Can you work these out from the model? Positions are in its coordinate system, mm. Face numbers are marked on the shaded views. A direction names the side the tool comes from. Round coordinates to 2 decimals unless told otherwise and drop trailing zeros. Loops run counter-clockwise (first coordinate to the right, second up) from the corner with the lowest first, then second, coordinate; pieces in that order, holes last. Notation, with made-up numbers: (51.5, 87) -> (81.5, 87) arc R22 ccw to (81.5, 106) -> close; hole circle Ø7 at (72.5, 9). An arc over 180 degrees is marked (long way). Write each question's results on one line, items separated by ' | '.
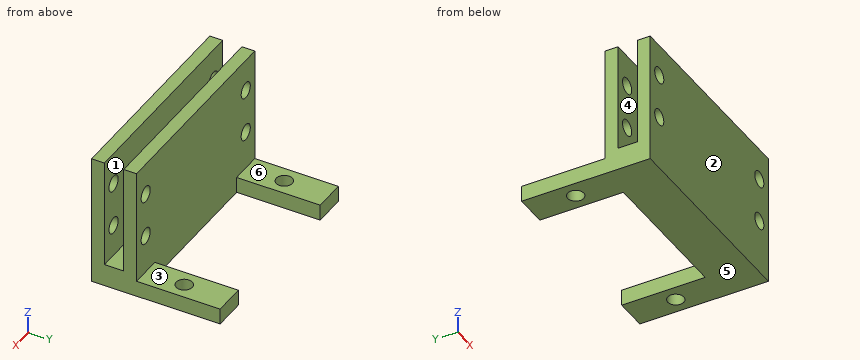
from build123d import *

# Parameters (mm, degrees)
SKETCH1_W               = 5
SKETCH1_H               = 13
SKETCH1_R               = 1.25
BOSS_EXTRUDE1_DEPTH     = 2.5
BOSS_EXTRUDE1_2_DEPTH   = 2.5
SKETCH1_5_W             = 32.5
SKETCH1_5_H             = 2
BOSS_EXTRUDE2_DEPTH     = 20.5
SKETCH1_6_W             = 32.5
SKETCH1_6_H             = 3
BOSS_EXTRUDE3_DEPTH     = 3.5
SKETCH2_R               = 1.25
CUT_EXTRUDE2_DEPTH      = 14
CUT_EXTRUDE2_DEPTH_BACK = 8


with BuildPart() as part:
    # Sketch1 → Boss-Extrude1 (new body)
    with BuildSketch(Plane.XY):
        with Locations((-13.75, 6.5)):
            Rectangle(SKETCH1_W, SKETCH1_H)
        with Locations((-13.75, 6)):
            Circle(SKETCH1_R, mode=Mode.SUBTRACT)
    extrude(amount=BOSS_EXTRUDE1_DEPTH)



with BuildPart() as body_2:
    # Sketch1 → Boss-Extrude1 2 (new body)
    with BuildSketch(Plane.XY):
        with Locations((13.75, 6.5)):
            Rectangle(SKETCH1_W, SKETCH1_H)
        with Locations((13.75, 6)):
            Circle(SKETCH1_R, mode=Mode.SUBTRACT)
    extrude(amount=BOSS_EXTRUDE1_2_DEPTH)


with BuildPart() as part_1:
    add(part.part)

    add(body_2.part)  # Boss-Extrude2 merges body 2
    # Sketch1<5> → Boss-Extrude2 (add)
    with BuildSketch(Plane.XY):
        with Locations((0, -1)):
            Rectangle(SKETCH1_5_W, SKETCH1_5_H)
        with Locations((0, -6)):
            Rectangle(SKETCH1_5_W, SKETCH1_5_H)
    extrude(amount=BOSS_EXTRUDE2_DEPTH)

    # Sketch1<6> → Boss-Extrude3 (add)
    with BuildSketch(Plane.XY):
        with Locations((0, -3.5)):
            Rectangle(SKETCH1_6_W, SKETCH1_6_H)
    extrude(amount=BOSS_EXTRUDE3_DEPTH)

    # Sketch2 → Cut-Extrude2 (cut, two sides)
    with BuildSketch(Plane(origin=(0, 0, 0), x_dir=(1, 0, 0), z_dir=(0, 1, 0))) as cut_extrude2_sk:
        with Locations((13.75, -8.5)):
            Circle(SKETCH2_R)
        with Locations((13.75, -15.5)):
            Circle(SKETCH2_R)
        with Locations((-13.75, -15.5)):
            Circle(SKETCH2_R)
        with Locations((-13.75, -8.5)):
            Circle(SKETCH2_R)
    extrude(amount=CUT_EXTRUDE2_DEPTH, mode=Mode.SUBTRACT)
    extrude(cut_extrude2_sk.sketch, amount=-CUT_EXTRUDE2_DEPTH_BACK, mode=Mode.SUBTRACT)


solid = part_1.part
1. Please list where these lines run through material, in increasing order: line 1 (Z direction, x = 13.75, y = -1); line 2 (Y direction, x = -8, z = 13.25); line 3 (Y direction, x = -13.75, z = 1). Write a range as from..to.
Final values:
line 1: 0..7.25, 9.75..14.25, 16.75..20.5 | line 2: -7..-5, -2..0 | line 3: -7..4.75, 7.25..13
2. If we section it at A-A (y = 9.75): List the corners of the cut face in (x, z) for me.
Final values:
outline: (-16.25, 0) -> (-11.25, 0) -> (-11.25, 2.5) -> (-16.25, 2.5) -> close; (11.25, 0) -> (16.25, 0) -> (16.25, 2.5) -> (11.25, 2.5) -> close
3. If we section it at C-C (x = 13.75): State how many separate pieces and enclosed holes the cut face has, then the cut area to 4 significant figures.
Final values:
separate pieces: 6 | enclosed holes: 0 | area: 98.75 mm2
4. We'd pull the mould along Y, two halves only. Please class the marked faces 1, 2, 3 and 4: pulls with the +Y half, pulls with the -Y half, needs draft (parallel to the pull), parting line crosses it, or undercut.
Final values:
face 1: undercut | face 2: pulls with the -Y half | face 3: needs draft | face 4: undercut
5. Will these pins go through, and if not, where does the flat tip stop? pin 1 (1 mm diameter, centred on x = 12.5, z = 5.5, fed in from +Y); pin 2 (1.5 mm diameter, centred on x = -14, y = 5, fed in from +Z); pin 3 (1.5 mm diameter, centred on x = 13.75, z = 15.5, fed in from -Y); pin 4 (0.9 mm diameter, centred on x = 2.5, y = -3, fed in from +Z).
Final values:
pin 1: y = 0 | pin 2: z = 2.5 | pin 3: through | pin 4: z = 3.5
6. If we section it at B-B (z = 6): List the corners of the cut face in (x, y) for me.
Final values:
outline: (-16.25, -7) -> (16.25, -7) -> (16.25, -5) -> (-16.25, -5) -> close; (-16.25, -2) -> (16.25, -2) -> (16.25, 0) -> (-16.25, 0) -> close
7. On a 3-axis mill with a long thin cutter (end or side, diameter ignored), from which of +Z, -Z, +X, -X, +Y, -Y can I reach the whole of each face in a straight line? I mean the marked faces 5 and 6. Say none if no direction works.
Final values:
face 5: -Z, +X, -X, +Y, -Y | face 6: +Z, +X, -X, +Y
8. If we section it at D-D (z = 8.5): List the corners of the cut face in (x, y) for me.
Final values:
outline: (-16.25, -7) -> (-15, -7) -> (-15, -5) -> (-16.25, -5) -> close; (-16.25, -2) -> (-15, -2) -> (-15, 0) -> (-16.25, 0) -> close; (-12.5, -7) -> (12.5, -7) -> (12.5, -5) -> (-12.5, -5) -> close; (-12.5, -2) -> (12.5, -2) -> (12.5, 0) -> (-12.5, 0) -> close; (15, -7) -> (16.25, -7) -> (16.25, -5) -> (15, -5) -> close; (15, -2) -> (16.25, -2) -> (16.25, 0) -> (15, 0) -> close
